Check sheet for the modelled part. Datum: model origin and axes. Units: mm. Face numbers are marked on the shaded views. A direction names the side the tool comes from. Coordinates: 2 decimals unless noted, no trailing zeros. Order: outer loops, then holes, each group sorted by start corner. A loop starts at its lowest first (then second) coordinate and runs counter-clockwise, first axis right, second up.
from build123d import *

# Parameters (mm, degrees)
SKETCH1_R           = 1.55
BOSS_EXTRUDE1_DEPTH = 7.5
FILLET2_R           = 1
SKETCH2_R           = 7
CUT_EXTRUDE1_DEPTH  = 10
SKETCH3_W           = 21.6
SKETCH3_H           = 38
SKETCH3_W_2         = 16
SKETCH3_H_2         = 32.4
BOSS_EXTRUDE9_DEPTH = 22
FILLET6_R           = 3


with BuildPart() as part:
    # Sketch1 → Boss-Extrude1 (new body)
    with BuildSketch(Plane(origin=(0, 0, 0), x_dir=(1, 0, 0), z_dir=(0, 1, 0))):
        with BuildLine():
            Line((-18, 20), (18, 20))
            ThreePointArc((18, 20), (19.414213562, 19.414213562), (20, 18))
            Line((20, 18), (20, -18))
            ThreePointArc((20, -18), (19.414213562, -19.414213562), (18, -20))
            Line((18, -20), (-18, -20))
            ThreePointArc((-18, -20), (-19.414213562, -19.414213562), (-20, -18))
            Line((-20, -18), (-20, 18))
            ThreePointArc((-20, 18), (-19.414213562, 19.414213562), (-18, 20))
        make_face()
        with Locations(Location((-17.22, 15.5, 0), (0, 0, 270))):
            Circle(SKETCH1_R, mode=Mode.SUBTRACT)
        with Locations(Location((-17.22, -15.5, 0), (0, 0, 270))):
            Circle(SKETCH1_R, mode=Mode.SUBTRACT)
        with Locations(Location((17.22, 15.5, 0), (0, 0, 270))):
            Circle(SKETCH1_R, mode=Mode.SUBTRACT)
        with Locations(Location((17.22, -15.5, 0), (0, 0, 270))):
            Circle(SKETCH1_R, mode=Mode.SUBTRACT)
    extrude(amount=BOSS_EXTRUDE1_DEPTH)

    # Fillet2
    fillet2_edges = [part.edges().sort_by_distance(p)[0] for p in [
        (0, 0, -20),
        (19.414213562, 0, -19.414213562),
        (20, 0, 0),
        (19.414213562, 0, 19.414213562),
        (19.414213562, 7.5, -19.414213562),
        (0, 7.5, -20),
        (-19.414213562, 7.5, -19.414213562),
        (-20, 7.5, 0),
        (-19.414213562, 7.5, 19.414213562),
        (0, 7.5, 20),
        (19.414213562, 7.5, 19.414213562),
        (0, 0, 20),
        (20, 7.5, 0),
        (-19.414213562, 0, 19.414213562),
        (-20, 0, 0),
        (-19.414213562, 0, -19.414213562),
    ]]
    fillet(fillet2_edges, radius=FILLET2_R)

    # Sketch2 → Cut-Extrude1 (cut)
    with BuildSketch(Plane(origin=(0, 7.5, 0), x_dir=(1, 0, 0), z_dir=(0, 1, 0))):
        with Locations(Location((0, 0, 0), (0, 0, 270))):
            Circle(SKETCH2_R)
    extrude(amount=-CUT_EXTRUDE1_DEPTH, mode=Mode.SUBTRACT)

    # Sketch3 → Boss-Extrude9 (add)
    with BuildSketch(Plane(origin=(0, 7.5, 0), x_dir=(1, 0, 0), z_dir=(0, 1, 0))):
        Rectangle(SKETCH3_W, SKETCH3_H)
        Rectangle(SKETCH3_W_2, SKETCH3_H_2, mode=Mode.SUBTRACT)
    extrude(amount=BOSS_EXTRUDE9_DEPTH)

    # Fillet6
    fillet6_edges = [part.edges().sort_by_distance(p)[0] for p in [
        (-10.8, 18.5, -19),
        (-10.8, 18.5, 19),
        (10.8, 18.5, 19),
        (10.8, 18.5, -19),
    ]]
    fillet(fillet6_edges, radius=FILLET6_R)


solid = part.part
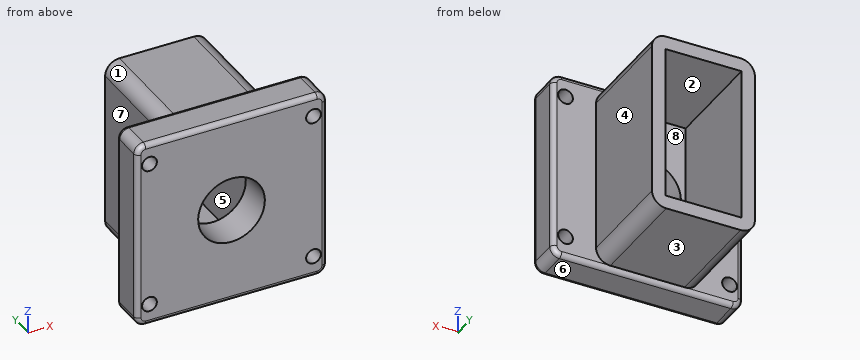
(1) Release check for a two-part mould opening along Z. For the marked faces 5, 6, 7 and 8 record: +Z half, -Z half, draft (parallel to the pull), parting line (faces both ways), or undercut.
Filled in:
face 5: undercut
face 6: -Z half
face 7: draft
face 8: undercut
(2) Thickness scan on probe 1 along X at (y, z) = (3.25, 15.5); probe 2 along Z at (x, y) = (0, 14.75); probe 3 along X at (y, z) = (17.25, -11). Record the ranges inside material, lowest first.
Filled in:
probe 1: x = -20 to -18.77, -15.67 to 15.67, 18.77 to 20
probe 2: z = -19 to -16.2, 16.2 to 19
probe 3: x = -10.8 to -8, 8 to 10.8
(3) Cross-section at A-A (x = 0). Enter the section's corners in (y, z), and give its area (3 significant figures).
Filled in:
outline: (0, -19) arc R1 ccw to (1, -20) - (6.5, -20) arc R1 ccw to (7.5, -19) - (29.5, -19) - (29.5, -16.2) - (7.5, -16.2) - (7.5, -7) - (0, -7) - close; (0, 7) - (7.5, 7) - (7.5, 16.2) - (29.5, 16.2) - (29.5, 19) - (7.5, 19) arc R1 ccw to (6.5, 20) - (1, 20) arc R1 ccw to (0, 19) - close
area: 317 mm2
(4) Go/stop test with flat-tipped pins: P1, Ø4.5, axis at x = -3.5, y = 18, coming from the -Z side; P2, Ø6.5, axis at y = 21, z = -6, coming from the -X side; P3, Ø4, axis at x = 17.22, z = -15.5, coming from the +Y side; P4, Ø12.5, axis at x = 0, z = 0, coming from the -Y side. Record where each tip stops, or that it passes through.
Filled in:
P1: stops at z = -19
P2: stops at x = -10.8
P3: stops at y = 7.5
P4: passes through
(5) Cross-section at C-C (x = 17.22). Enter the section's corners in (y, z), and give its area (3 significant figures).
Filled in:
outline: (0, -19) arc R1 ccw to (1, -20) - (6.5, -20) arc R1 ccw to (7.5, -19) - (7.5, -17.05) - (0, -17.05) - close; (0, -13.95) - (7.5, -13.95) - (7.5, 13.95) - (0, 13.95) - close; (0, 17.05) - (7.5, 17.05) - (7.5, 19) arc R1 ccw to (6.5, 20) - (1, 20) arc R1 ccw to (0, 19) - close
area: 253 mm2
(6) Cross-section at D-D (y = 22.5). Enter the section's corners in (x, z), and give its area (3 significant figures).
Filled in:
outline: (-10.8, -16) arc R3 ccw to (-7.8, -19) - (7.8, -19) arc R3 ccw to (10.8, -16) - (10.8, 16) arc R3 ccw to (7.8, 19) - (-7.8, 19) arc R3 ccw to (-10.8, 16) - close; hole (-8, -16.2) - (8, -16.2) - (8, 16.2) - (-8, 16.2) - close
area: 295 mm2
(7) Tool access check on the marked faces 1, 2, 3 and 4. Record the directions out of +Z, -Z, +X, -X, +Y, -Y that give a thin tool (end or side, any length) a straight path to the whole face; none if there is none.
Filled in:
face 1: +Z, -X, +Y
face 2: +Y
face 3: -Z, +X, -X, +Y
face 4: +Z, -Z, +X, +Y
(8) Cross-section at B-B (z = 0). Enter the section's corners in (x, y).
Filled in:
outline: (-20, 1) arc R1 ccw to (-19, 0) - (-7, 0) - (-7, 7.5) - (-8, 7.5) - (-8, 29.5) - (-10.8, 29.5) - (-10.8, 7.5) - (-19, 7.5) arc R1 ccw to (-20, 6.5) - close; (7, 0) - (19, 0) arc R1 ccw to (20, 1) - (20, 6.5) arc R1 ccw to (19, 7.5) - (10.8, 7.5) - (10.8, 29.5) - (8, 29.5) - (8, 7.5) - (7, 7.5) - close
